Autodesk Inventor part; units mm, degrees
ref_plane "YZ Plane" through (0, 0, 0) normal (1, 0, 0) x (0, 1, 0)
ref_plane "XZ Plane" through (0, 0, 0) normal (0, 1, 0) x (-1, 0, 0)
ref_plane "XY Plane" through (0, 0, 0) normal (0, 0, 1) x (1, 0, 0)
sketch "Sketch1" plane through (0, 0, 0) normal (0, 1, 0) x (-1, 0, 0)
  circle A0 centre (0, 0) radius 6.6
  dimension "d0" = 13.2
extrude "Extrusion1" add sketch "Sketch1" along normal blind 20
sketch "Sketch3" plane through (0, 20, 0) normal (0, 1, 0) x (1, 0, 0)
  circle A0 centre (0, 0) radius 40
  dimension "d4" = 80
extrude "Extrusion2" add sketch "Sketch3" along normal blind 140
sketch "Sketch4" plane through (0, 160, 0) normal (0, 1, 0) x (1, 0, 0)
  circle A0 centre (0, 0) radius 36
  circle A1 centre (0, 0) radius 40
  dimension "d7" = 72
extrude "Extrusion3" cut sketch "Sketch4" against normal blind 130 contours A0
sketch "Sketch5" plane through (0, 0, 0) normal (0, -1, 0) x (1, 0, 0)
  circle A0 centre (0, 0) radius 5.3852
  circle A1 centre (0, 0) radius 6.6
extrude "Extrusion4" cut sketch "Sketch5" against normal blind 130 contours A0
sketch "Sketch6" plane through (0, 160, 0) normal (0, 1, 0) x (1, 0, 0)
  line L0 (23, -36) -> (-22, -36)
  line L1 (-22, -36) -> (-22, -48)
  line L2 (-22, -48) -> (23, -48)
  line L3 (23, -48) -> (23, -36)
  point P0 (0, 0)
extrude "Extrusion5" add sketch "Sketch6" against normal blind 130
sketch "Sketch7" plane through (0, 30, 0) normal (0, -1, 0) x (1, 0, 0)
  line L0 (-25, 44) -> (25, 44)
  line L1 (25, 44) -> (25, 40)
  line L2 (25, 40) -> (-25, 40)
  line L3 (-25, 40) -> (-25, 44)
  line L4 (23, 48) -> (-22, 48)
  point P0 (0, 0)
  dimension "d17" = 4
extrude "Extrusion6" cut sketch "Sketch7" against normal blind 60
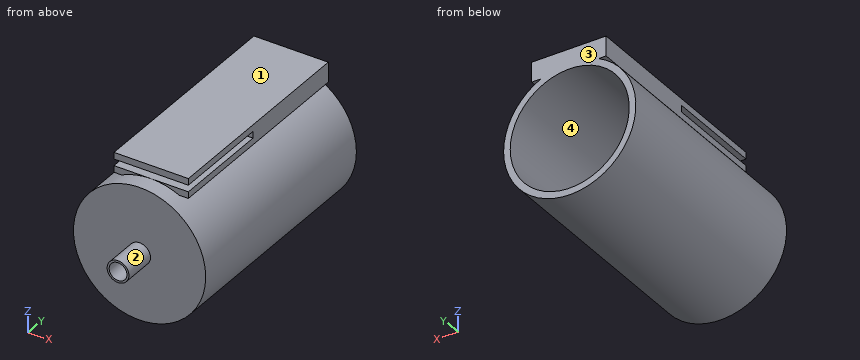
Here's how the part is built. I have some questions about the finished solid (model axes, mm). Face numbers are marked on the shaded views. Round coordinates to 2 decimals unless told otherwise and drop trailing zeros. Order: outer loops, then holes, each group sorted by start corner. A loop starts at its lowest first (then second) coordinate and runs counter-clockwise, first axis right, second up. Notation, with made-up numbers: M 79.25,53 L 115.25,53 A28 cw 115.25,76 Z; hole C 9,24 d3. An arc over 180 degrees is marked long. Use CSV: the item, a comma, the result in double quotes.
1) I want a section at B-B (y = 130). List the corners of the cut face in (x, z) for me.
Taken from the geometry:
outline,"M -22,36 L -17.44,36 A40 ccw long 17.44,36 L 23,36 L 23,48 L -22,48 Z; hole C 0,0 d72"
2) I want a section at C-C (z = 0). List the corners of the cut face in (x, y) for me, then the cut area to 3 significant figures.
Taken from the geometry:
outline,"M -40,20 L -6.6,20 L -6.6,0 L -5.39,0 L -5.39,30 L -36,30 L -36,160 L -40,160 Z; M 5.39,0 L 6.6,0 L 6.6,20 L 40,20 L 40,160 L 36,160 L 36,30 L 5.39,30 Z"
area,"1,780 mm^2"
3) I want a section at A-A (y = 66.5). List the corners of the cut face in (x, z) for me, then the cut area to 3 significant figures.
Taken from the geometry:
outline,"M -22,36 L -17.44,36 A40 ccw long 17.44,36 L 23,36 L 23,40 L -22,40 Z; M -22,44 L 23,44 L 23,48 L -22,48 Z; hole C 0,0 d72"
area,"1,220 mm^2"
4) I need wall thicknesses on line 1 along Z through (x, y) = (0, 121); line 2 along Z through (x, y) = (0, 9); line 3 along Z through (x, y) = (0, 60.5). Which ranges of each line are inside material? Lowest first, please. Write a range as [from, to].
Taken from the geometry:
line 1,"[-40, -36], [36, 48]"
line 2,"[-6.6, -5.39], [5.39, 6.6]"
line 3,"[-40, -36], [36, 40], [44, 48]"
5) I'm going to push flat-ended pins straight in: P1, Ø5, axis at x = -30, z = 0, coming from the -Y side; P2, Ø10, axis at x = -13.5, z = 0.5, coming from the +Y side; P3, Ø13, axis at y = 111.5, z = 43, coming from the +X side. Where does each tip first touch, or does it pass through?
Taken from the geometry:
P1,"y = 20"
P2,"y = 30"
P3,"x = 23"
6) If we mould it in two halves opening along Z, with no side actions, what happens to the marked faces 1, 2, 3 and 4? For each: pulls with the +Z half, pulls with the -Z half, needs draft (parallel to the pull), parting line crosses it, or undercut.
Taken from the geometry:
face 1,"pulls with the +Z half"
face 2,"parting line crosses it"
face 3,"needs draft"
face 4,"undercut"
7) I want a section at D-D (z = 14). List the corners of the cut face in (x, y) for me.
Taken from the geometry:
outline,"M -37.47,20 L 37.47,20 L 37.47,160 L 33.17,160 L 33.17,30 L -33.17,30 L -33.17,160 L -37.47,160 Z"
